```python
from build123d import *

# Parameters (mm, degrees)
EXTRUDE1_DEPTH     = 364.33125
SKETCH2_R          = 1.5875
CUT_EXTRUDE1_DEPTH = 1.524


with BuildPart() as part:
    # Sketch1 → Extrude1 (new body, symmetric)
    with BuildSketch(Plane.XY):
        Polygon((58.674, 15.6718), (58.674, -15.6718), (57.15, -15.6718), (57.15, -0.762), (44.45, -0.762), (44.45, -7.7851), (42.926, -7.7851), (42.926, 7.7851), (44.45, 7.7851), (44.45, 0.762), (57.15, 0.762), (57.15, 15.6718), align=None)
    extrude(amount=EXTRUDE1_DEPTH, both=True)

    # Sketch2 → Cut-Extrude1 (cut)
    with BuildSketch(Plane.ZY.offset(-57.15)):
        with Locations((357.98125, -11.72845)):
            Circle(SKETCH2_R)
        with Locations((-357.98125, -11.72845)):
            Circle(SKETCH2_R)
    extrude(amount=-CUT_EXTRUDE1_DEPTH, mode=Mode.SUBTRACT)


solid = part.part
```
The listing builds one solid part. Answer for the finished solid, in the listing's coordinates (mm). A direction names the side the tool comes from. Round coordinates to 2 decimals unless told otherwise and drop trailing zeros. Write each loop counter-clockwise with the first axis right and the second up, starting at its lowest first coordinate (ties: lowest second). Pieces come first, ordered by that corner, then holes. Notation, with made-up numbers: (6.25, 33) -> (55.25, 33) arc R27 ccw to (55.25, 71) -> close; hole circle Ø10 at (89, -14). An arc over 180 degrees is marked (long way). Use CSV: the item, a comma, the result in double quotes. Start each with the question number.
(1) Section A-A on z = 315 is taken. Give the vertices of the cut face in (x, y), then the cut area to 3 significant figures.
(2) Section B-B on x = 50 is taken. Give the vertices of the cut face in (y, z), then the cut area to 3 significant figures.
(3) The mould has two halves that part along X. Classify faces 4 (the face through (53, 0, 364.331)), 5 (the face through (42.926, 0, 5)), 6 (the face through (51, -0.762, 5)): released by +X, released by -X, zero draft, split by the parting line, or undercut.
(4) Which of the six approach directions +Z, -Z, +X, -X, +Y, -Y give full straight-line access (tool end or side, diameter ignored) to faces 1 (the face through (53, 0, -364.331)), 2 (the face through (57.15, -8, 5)), 3 (the face through (57.15, 8, 5))?
(5) Consider L1, parallel to X at y = 1.5, z = -33.5; L2, parallel to Y at x = 48.25, z = -244; L3, parallel to X at y = 13, z = -184. Determine where each line is inside the solid, lowest interval first. Write a range as from..to.
(6) Each of these flat-tipped pins is pushed along its axis until it touches: pin 1 (4 mm diameter, centred on x = 47.5, z = -284, fed in from +Y); pin 2 (1.5 mm diameter, centred on x = 49, y = 3.5, fed in from -Z); pin 3 (0.5 mm diameter, centred on x = 43.5, z = 25, fed in from +Y); pin 4 (4 mm diameter, centred on y = -11.73, z = 357.98, fed in from -X). Where does it stop, or does it pass through?
A:
1,outline,"(42.93, -7.79) -> (44.45, -7.79) -> (44.45, -0.76) -> (57.15, -0.76) -> (57.15, -15.67) -> (58.67, -15.67) -> (58.67, 15.67) -> (57.15, 15.67) -> (57.15, 0.76) -> (44.45, 0.76) -> (44.45, 7.79) -> (42.93, 7.79) -> close"
1,area,"90.9 mm²"
2,outline,"(-0.76, -364.33) -> (0.76, -364.33) -> (0.76, 364.33) -> (-0.76, 364.33) -> close"
2,area,"1,110 mm²"
3,face 4,"zero draft"
3,face 5,"released by -X"
3,face 6,"undercut"
4,face 1,"-Z, +X, -X, +Y, -Y"
4,face 2,"+Z, -Z, -Y"
4,face 3,"+Z, -Z, +Y"
5,L1,"x = 42.93..44.45, 57.15..58.67"
5,L2,"y = -0.76..0.76"
5,L3,"x = 57.15..58.67"
6,pin 1,"stops at y = 0.76"
6,pin 2,"passes through"
6,pin 3,"stops at y = 7.79"
6,pin 4,"stops at x = 57.15"
